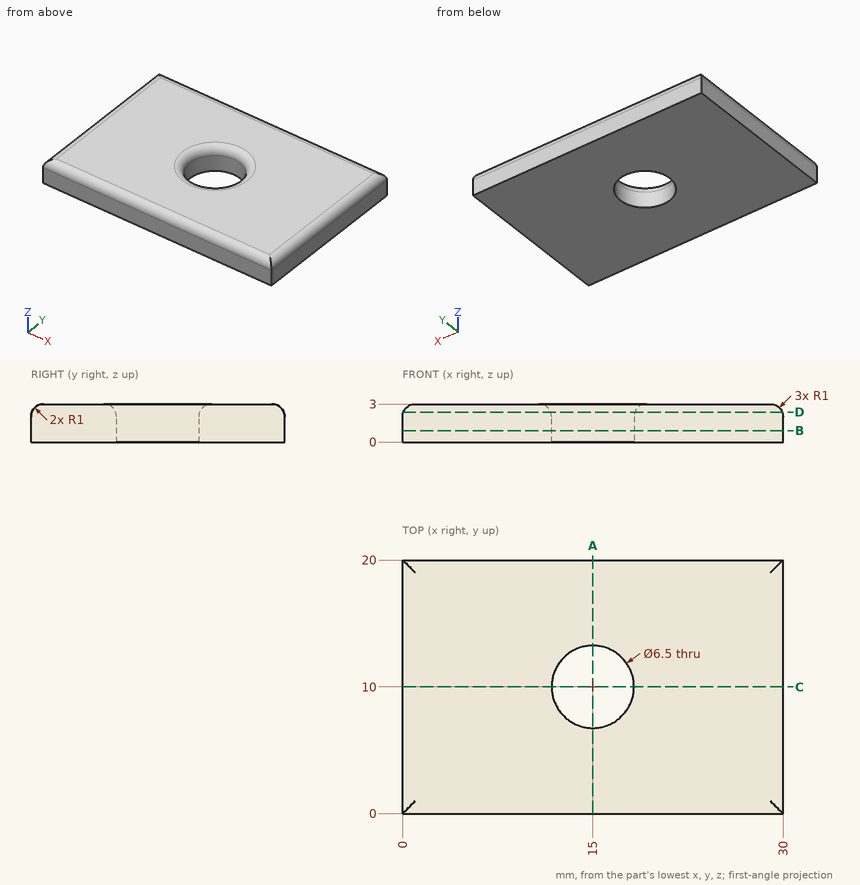
Geometry: see drawing. Coordinates: mm, zero at the bounding-box minimum. Coordinates: 2 decimals unless noted, no trailing zeros. Order: outer loops, then holes, each group sorted by start corner. A loop starts at its lowest first (then second) coordinate and runs counter-clockwise, first axis right, second up. Notation, with made-up numbers: (-6.5, 70) -> (41.5, 70) arc R16 cw to (41.5, 90) -> close; hole circle Ø5 at (19, -31.5). An arc over 180 degrees is marked (long way). Write each question's results on one line, items separated by ' | '. Start each with the question number.
1) Cut plane C-C, the plane y = 10. Output: boundary loops of the cut face in (x, z).
2) Cut plane D-D, the plane z = 2.35. Output: boundary loops of the cut face in (x, y), and give its area (3 significant figures).
3) First-contact query: pin 1 (4 mm diameter, centred on x = 15, y = 10, fed in from +Z). Flat tip, straight axial feed; report the tip coordinate or a pass-through.
4) Cut plane B-B, the plane z = 0.9. Output: boundary loops of the cut face in (x, y), and give its area (3 significant figures).
5) Material intervals for line 1 along Y through (x, z) = (15, 0.75); line 2 along X through (y, z) = (11.25, 0.1); line 3 along X through (y, z) = (4.75, 2.1), sorted ascending.
6) Cut plane A-A, the plane x = 15. Output: boundary loops of the cut face in (y, z).
Checks:
1) outline: (0, 0) -> (11.75, 0) -> (11.75, 2) arc R1 ccw to (10.75, 3) -> (1, 3) arc R1 ccw to (0, 2) -> close; (18.25, 0) -> (30, 0) -> (30, 2) arc R1 ccw to (29, 3) -> (19.25, 3) arc R1 ccw to (18.25, 2) -> close
2) outline: (0.06, 0.06) -> (29.94, 0.06) -> (29.94, 19.94) -> (0.06, 19.94) -> close; hole circle Ø6.63 at (15, 10) | area: 559 mm^2
3) pin 1: through
4) outline: (0, 0) -> (30, 0) -> (30, 20) -> (0, 20) -> close; hole circle Ø6.5 at (15, 10) | area: 567 mm^2
5) line 1: 0 to 6.75, 13.25 to 20 | line 2: 0 to 12, 18 to 30 | line 3: 0.01 to 29.99
6) outline: (0, 0) -> (6.75, 0) -> (6.75, 2) arc R1 ccw to (5.75, 3) -> (1, 3) arc R1 ccw to (0, 2) -> close; (13.25, 0) -> (20, 0) -> (20, 2) arc R1 ccw to (19, 3) -> (14.25, 3) arc R1 ccw to (13.25, 2) -> close
